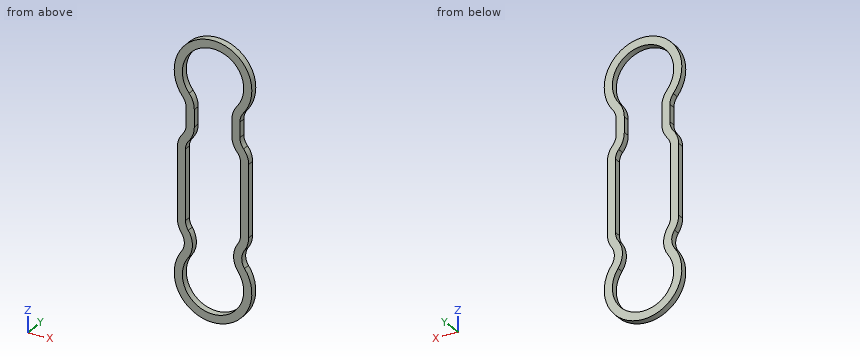
Autodesk Inventor part; units mm, degrees
ref_plane "YZ Plane" through (0, 0, 0) normal (1, 0, 0) x (0, 1, 0)
ref_plane "XZ Plane" through (0, 0, 0) normal (0, 1, 0) x (-1, 0, 0)
ref_plane "XY Plane" through (0, 0, 0) normal (0, 0, 1) x (1, 0, 0)
sketch "Sketch1" plane through (0, 0, 0) normal (0, 1, 0) x (-1, 0, 0)
  line L0 (13.9, 33.875) -> (-13.9, 33.875)
  line L1 (-13.9, 33.875) -> (-13.9, -33.875)
  line L2 (-13.9, -33.875) -> (13.9, -33.875)
  line L3 (13.9, -33.875) -> (13.9, 33.875)
  circle A0 centre (9.4, 30.5) radius 1.7
  circle A1 centre (-9.4, 15) radius 1.7
  circle A2 centre (9.4, -15) radius 1.7
  circle A3 centre (-9.4, -15) radius 1.7
  circle A4 centre (-9.4, -30.5) radius 1.7
  circle A5 centre (9.4, -30.5) radius 1.7
  circle A6 centre (9.4, 15) radius 1.7
  circle A7 centre (-9.4, 30.5) radius 1.7
  arc A8 (-3.4662, -17.8593) -> (3.4662, -17.8593) centre (0, -22) ccw
  line L4 (4.7, 5.1) -> (4.7, -10.1)
  arc A9 (2.75, -12.0994) -> (4.7, -10.1) centre (2.7, -10.1) ccw
  arc A10 (-4.7, -10.1) -> (-2.75, -12.0994) centre (-2.7, -10.1) ccw
  line L5 (-4.7, -10.1) -> (-4.7, 5.1)
  line L6 (-2.75, 7.0994) -> (-2.75, 16.3257)
  arc A11 (3.4662, 17.8593) -> (-3.4662, 17.8593) centre (0, 22) ccw
  line L7 (2.75, -12.0994) -> (2.75, -16.3257)
  arc A12 (-5.2039, -18.2745) -> (5.2039, -18.2745) centre (0, -22) ccw
  line L8 (-3.75, 14.4782) -> (-3.75, 11.1034)
  arc A13 (-5.0936, 7.4643) -> (-5.7, 5.8219) centre (-3.1726, 5.8219) ccw
  arc A14 (-5.7, -10.1) -> (-5.1619, -11.8144) centre (-2.7, -10.1) ccw
  arc A15 (5.1619, -11.8144) -> (5.7, -10.1001) centre (2.7, -10.1) ccw
  line L9 (5.7, -10.1001) -> (5.7004, 5.4185)
  arc A16 (5.7004, 5.4185) -> (5.0937, 7.0617) centre (3.1718, 5.4185) ccw
  line L10 (3.75, 10.7009) -> (3.75, 14.4782)
  arc A17 (4.9867, 17.9884) -> (-4.9867, 17.9884) centre (0, 22) ccw
  line L11 (-6.35, 14.4782) -> (-6.35, 11.1034)
  arc A18 (-7.0698, 9.1539) -> (-8.3, 5.8219) centre (-3.1726, 5.8219) ccw
  line L12 (-8.3, 5.8219) -> (-8.3, -10.1)
  arc A19 (-8.3, -10.1) -> (-7.2955, -13.3003) centre (-2.7, -10.1) ccw
  arc A20 (-7.318, -16.761) -> (7.318, -16.761) centre (0, -22) ccw
  arc A21 (7.2955, -13.3003) -> (8.3, -10.1) centre (2.7, -10.1) ccw
  line L13 (8.3, -10.1) -> (8.3, 5.4787)
  arc A22 (8.3, 5.4787) -> (7.0698, 8.7513) centre (3.1718, 5.4185) ccw
  line L14 (6.35, 10.7009) -> (6.35, 14.4782)
  arc A23 (7.0125, 16.3586) -> (-7.0125, 16.3586) centre (0, 22) ccw
  arc A24 (-7.318, -16.761) -> (-7.2955, -13.3003) centre (-9.7573, -15.0147) ccw
  arc A25 (7.2955, -13.3003) -> (7.318, -16.761) centre (9.7573, -15.0147) ccw
  arc A26 (-7.0698, 9.1539) -> (-6.35, 11.1034) centre (-9.35, 11.1034) ccw
  arc A27 (-6.35, 14.4782) -> (-7.0125, 16.3586) centre (-9.35, 14.4782) ccw
  arc A28 (7.0125, 16.3586) -> (6.35, 14.4782) centre (9.35, 14.4782) ccw
  arc A29 (6.35, 10.7009) -> (7.0698, 8.7513) centre (9.35, 10.7009) ccw
  line L15 (-5.7, -10.1) -> (-5.7, 5.8219)
  arc A30 (-5.0936, 7.4643) -> (-5.7, 5.8219) centre (-3.1726, 5.8219) ccw
  arc A31 (-5.0936, 7.4643) -> (-3.75, 11.1034) centre (-9.35, 11.1034) ccw
  line L16 (-3.75, 11.1034) -> (-3.75, 14.4782)
  arc A32 (-3.75, 14.4782) -> (-4.9867, 17.9884) centre (-9.35, 14.4782) ccw
  arc A33 (4.9867, 17.9884) -> (-4.9867, 17.9884) centre (0, 22) ccw
  arc A34 (4.9867, 17.9884) -> (3.75, 14.4782) centre (9.35, 14.4782) ccw
  line L17 (3.75, 14.4782) -> (3.75, 10.7009)
  arc A35 (3.75, 10.7009) -> (5.0937, 7.0617) centre (9.35, 10.7009) ccw
  arc A36 (5.7004, 5.4185) -> (5.0937, 7.0617) centre (3.1718, 5.4185) ccw
  arc A37 (5.1619, -11.8144) -> (5.7, -10.1001) centre (2.7, -10.1) ccw
  arc A38 (5.1619, -11.8144) -> (5.2039, -18.2745) centre (9.7573, -15.0147) ccw
  arc A39 (-5.2039, -18.2745) -> (5.2039, -18.2745) centre (0, -22) ccw
  arc A40 (-5.2039, -18.2745) -> (-5.1619, -11.8144) centre (-9.7573, -15.0147) ccw
  arc A41 (-5.7, -10.1) -> (-5.1619, -11.8144) centre (-2.7, -10.1) ccw
  line L18 (2.75, 16.3257) -> (2.75, 7.0994)
  line L19 (-2.75, -16.3257) -> (-2.75, -12.0994)
  arc A42 (-3.4662, -17.8593) -> (-2.75, -16.3257) centre (-4.75, -16.3257) ccw
  arc A43 (-2.75, 16.3257) -> (-3.4662, 17.8593) centre (-4.75, 16.3257) ccw
  arc A44 (3.4662, 17.8593) -> (2.75, 16.3257) centre (4.75, 16.3257) ccw
  arc A45 (2.75, -16.3257) -> (3.4662, -17.8593) centre (4.75, -16.3257) ccw
  arc A46 (-2.75, 7.0994) -> (-4.7, 5.1) centre (-2.7, 5.1) ccw
  arc A47 (4.7, 5.1) -> (2.75, 7.0994) centre (2.7, 5.1) ccw
  line L20 (0, -33.875) -> (0, 33.875) construction
  arc A48 (-5.95, 14.4782) -> (-6.7008, 16.6094) centre (-9.35, 14.4782) ccw
  line L21 (-5.95, 14.4782) -> (-5.95, 11.1034)
  arc A49 (-6.7658, 8.894) -> (-5.95, 11.1034) centre (-9.35, 11.1034) ccw
  arc A50 (-6.7658, 8.894) -> (-7.9, 5.8219) centre (-3.1726, 5.8219) ccw
  line L22 (-7.9, 5.8219) -> (-7.9, -10.1)
  arc A51 (-7.9, -10.1) -> (-6.9672, -13.0717) centre (-2.7, -10.1) ccw
  arc A52 (-6.9928, -16.9939) -> (-6.9672, -13.0717) centre (-9.7573, -15.0147) ccw
  arc A53 (-6.9928, -16.9939) -> (6.9928, -16.9939) centre (0, -22) ccw
  arc A54 (6.9672, -13.0717) -> (6.9928, -16.9939) centre (9.7573, -15.0147) ccw
  arc A55 (6.9672, -13.0717) -> (7.9, -10.1) centre (2.7, -10.1) ccw
  line L23 (7.9, -10.1) -> (7.9, 5.4763)
  arc A56 (7.9, 5.4763) -> (6.7658, 8.4914) centre (3.1718, 5.4185) ccw
  arc A57 (5.95, 10.7009) -> (6.7658, 8.4914) centre (9.35, 10.7009) ccw
  line L24 (5.95, 10.7009) -> (5.95, 14.4782)
  arc A58 (6.7008, 16.6094) -> (5.95, 14.4782) centre (9.35, 14.4782) ccw
  arc A59 (6.7008, 16.6094) -> (-6.7008, 16.6094) centre (0, 22) ccw
  arc A60 (5.2983, 17.7376) -> (-5.2983, 17.7376) centre (0, 22) ccw
  arc A61 (5.2983, 17.7376) -> (4.15, 14.4782) centre (9.35, 14.4782) ccw
  line L25 (4.15, 10.7009) -> (4.15, 14.4782)
  arc A62 (4.15, 10.7009) -> (5.3977, 7.3216) centre (9.35, 10.7009) ccw
  arc A63 (6.1004, 5.4185) -> (5.3977, 7.3216) centre (3.1718, 5.4185) ccw
  line L26 (6.1004, 5.4185) -> (6.1, -10.1001)
  arc A64 (5.4901, -12.043) -> (6.1, -10.1001) centre (2.7, -10.1) ccw
  arc A65 (5.4901, -12.043) -> (5.5292, -18.0417) centre (9.7573, -15.0147) ccw
  arc A66 (-5.5292, -18.0417) -> (5.5292, -18.0417) centre (0, -22) ccw
  arc A67 (-5.5292, -18.0417) -> (-5.4901, -12.043) centre (-9.7573, -15.0147) ccw
  arc A68 (-6.1, -10.1) -> (-5.4901, -12.043) centre (-2.7, -10.1) ccw
  line L27 (-6.1, -10.1) -> (-6.1, 5.8219)
  arc A69 (-5.3976, 7.7242) -> (-6.1, 5.8219) centre (-3.1726, 5.8219) ccw
  arc A70 (-5.3976, 7.7242) -> (-4.15, 11.1034) centre (-9.35, 11.1034) ccw
  line L28 (-4.15, 14.4782) -> (-4.15, 11.1034)
  arc A71 (-4.15, 14.4782) -> (-5.2983, 17.7376) centre (-9.35, 14.4782) ccw
  point P0 (0, 0)
  point P1 (0, 0)
  point P2 (-6.35, 15.6221)
  point P3 (-6.35, 9.8461)
  point P4 (6.35, 9.4436)
  point P5 (6.35, 15.6221)
  point P6 (-7.3624, -13.3004)
  point P7 (-5.7039, -14.8852)
  point P8 (-5.7004, -15.0354)
  point P9 (-7.2703, -16.695)
  point P10 (7.2703, -16.695)
  point P11 (5.7004, -15.0354)
  point P12 (5.7039, -14.8852)
  point P13 (7.3624, -13.3004)
  point P14 (6.35, 13.663)
  point P15 (7.2703, 16.695)
  point P16 (-7.2703, 16.695)
  point P17 (-6.35, 13.663)
  point P18 (-5.7, 5.8219)
  point P19 (5.3977, 7.3216)
  point P20 (5.5292, -18.0417)
  point P21 (-5.4901, -12.043)
  point P22 (-5.2983, 17.7376)
  point P23 (4.15, 14.4782)
  dimension "d0" = 1
  dimension "d1" = 1
  dimension "d2" = 3
  dimension "d3" = 2.6
  dimension "d4" = 8.3
  dimension "d5" = 1
  dimension "d6" = 0.4
  dimension "d7" = 0.4
  dimension "d8" = 0.4
  dimension "d9" = 0.4
  dimension "d10" = 0.4
  dimension "d11" = 0.4
  dimension "d12" = 0.4
  dimension "d13" = 0.4
  dimension "d14" = 0.4
  dimension "d15" = 0.4
  dimension "d16" = 0.4
  dimension "d17" = 0.4
  dimension "d18" = 0.4
  dimension "d19" = 0.4
  dimension "d20" = 0.4
extrude "Extrusion1" add sketch "Sketch1" along normal blind 1.5 contours A48 A59 A58 L24 A57 A56 L23 A55 A54 A53 A52 A51 L22 A50 A49 L21
properties part number "Base Seal"
Source: CAD feature listing. Evaluate the final solid. Frame: model axes, mm. Round coordinates to 2 decimals unless told otherwise and drop trailing zeros. Loops run counter-clockwise (first coordinate to the right, second up) from the corner with the lowest first, then second, coordinate; pieces in that order, holes last. Notation, with made-up numbers: M 22.5,-12.5 L 65.5,-12.5 A10 cw 65.5,0.5 Z; hole C 72.5,75 d3. An arc over 180 degrees is marked long. Use a Markdown table: item, result. Add a question column.
1. Section query A-A on x = 0. Return the cut outline in (y, z).
2. Contact query for flat-ended pins moving along their axis: P1, Ø0.8, axis at y = 1, z = -4.5, coming from the -X side; P2, Ø6, axis at x = -3, z = -1.5, coming from the -Y side. Output: stop coordinate, or through.
3. Line query: line 1 (X direction, y = 1.15, z = 22); line 2 (Z direction, x = -7, y = 0.1); line 3 (X direction, y = 0.1, z = 12). Output: solid intervals per line, ascending.
4. Section query B-B on z = 22. Return the cut outline in (x, y).
Reported:
| question | item | result |
|---|---|---|
| 1 | outline | M 0,-30.6 L 1.5,-30.6 L 1.5,-28.8 L 0,-28.8 Z; M 0,28.8 L 1.5,28.8 L 1.5,30.6 L 0,30.6 Z |
| 2 | P1 | stops at x = -7.9 |
| 2 | P2 | passes through |
| 3 | line 1 | x = -8.6 to -6.8, 6.8 to 8.6 |
| 3 | line 2 | z = -27 to -17, -13.02 to 8.19, 17 to 27 |
| 3 | line 3 | x = -5.95 to -4.15, 4.15 to 5.95 |
| 4 | outline | M -8.6,0 L -6.8,0 L -6.8,1.5 L -8.6,1.5 Z; M 6.8,0 L 8.6,0 L 8.6,1.5 L 6.8,1.5 Z |
